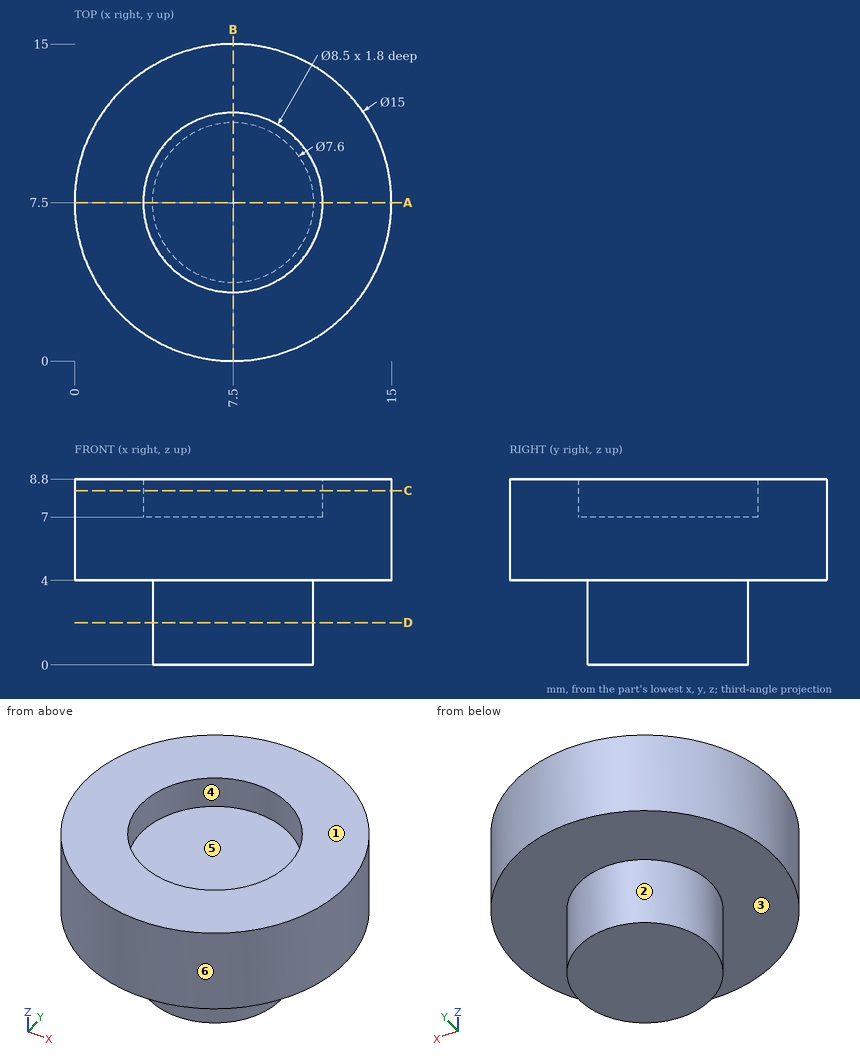
Can you work these out from the drawing? Everything is in mm from the part's minimum corner. A direction names the side the tool comes from. Give positions to 0.01 mm unless a question says otherwise; leave off trailing zeros. Loops run counter-clockwise (first coordinate to the right, second up) from the corner with the lowest first, then second, coordinate; pieces in that order, holes last. Notation, with made-up numbers: M 83,-10 L 105,-10 A14 ccw 105,-4 Z; hole C -29,57 d6. An arc over 180 degrees is marked long. Put each result on its own line as item: value. Start each with the question number.
(1) If we mould it in two halves opening along X, with no side actions, what happens to the marked faces 3, 4, 5 and 6? For each: +X half, -X half, draft (parallel to the pull), parting line (faces both ways), or undercut.
(2) I want a section at C-C on z = 8.25. Please give me the cut outline in (x, y), then the cut area to 3 significant figures.
(3) Will these pins go through, and if not, where does the flat tip stop? pin 1 Ø3 at (x, z) = (7.5, 1.5) entering from -Y; pin 2 Ø4 at (x, z) = (10, 1) entering from +Y; pin 3 Ø1 at (y, z) = (3.5, 6.5) entering from +X.
(4) I need wall thicknesses on line 1 along Y through (x, z) = (7.5, 7.9); line 2 along Z through (x, y) = (7, 13.5); line 3 along X through (y, z) = (8.75, 7.25). Which ranges of each line are inside material? Lowest first, please. Write a range as [from, to].
(5) I want a section at D-D on z = 2. Please give me the cut outline in (x, y), then the cut area to 3 significant figures.
(6) I want a section at A-A on y = 7.5. Please give me the cut outline in (x, z).
(7) For the marked faces 1 and 2, which set-ups out of +Z, -Z, +X, -X, +Y, -Y let a thin tool reach every point of the face, with its end or its side?
Answer block:
1. face 3: draft
1. face 4: undercut
1. face 5: undercut
1. face 6: parting line
2. outline: C 7.5,7.5 d15; hole C 7.5,7.5 d8.5
2. area: 120 mm^2
3. pin 1: y = 3.7
3. pin 2: y = 11.27
3. pin 3: x = 14.13
4. line 1: [0, 3.25], [11.75, 15]
4. line 2: [4, 8.8]
4. line 3: [0.1, 3.44], [11.56, 14.9]
5. outline: C 7.5,7.5 d7.6
5. area: 45.4 mm^2
6. outline: M 0,4 L 3.7,4 L 3.7,0 L 11.3,0 L 11.3,4 L 15,4 L 15,8.8 L 11.75,8.8 L 11.75,7 L 3.25,7 L 3.25,8.8 L 0,8.8 Z
7. face 1: +Z, +X, -X, +Y, -Y
7. face 2: -Z
